Verification items for the finished model (mm, model axes). Face numbers are marked on the shaded views. A direction names the side the tool comes from. Coordinates: 2 decimals unless noted, no trailing zeros. Order: outer loops, then holes, each group sorted by start corner. A loop starts at its lowest first (then second) coordinate and runs counter-clockwise, first axis right, second up.
Q1. Thickness scan on line 1 (Z direction, x = 14, y = 31.5); line 2 (Y direction, x = 5.5, z = -31); line 3 (Z direction, x = 36, y = -1). Record the ranges inside material, lowest first.
Q2. Set-up check for the marked faces 4 and 5: record each of +Z, -Z, +X, -X, +Y, -Y from which the full face is reachable in a straight line by a thin tool's end or side.
Q3. Draft check along Y on the marked faces 1, 2 and 3. Enter one of: pulls with the +Y half, pulls with the -Y half, needs draft (parallel to the pull), parting line crosses it, or undercut.
Q4. Depth check by flat-ended pin: P1, Ø4.5, axis at x = 2.5, z = -9.5, coming from the +Y side; P2, Ø3, axis at x = 26.5, z = 12.5, coming from the +Y side; P3, Ø4, axis at y = 28.5, z = 12.5, coming from the +X side. Enter the tip coordinate at first touch or a pass-through.
Q5. Cross-section at A-A, the plane z = -4. Record the boundary of the cut face in (x, y).
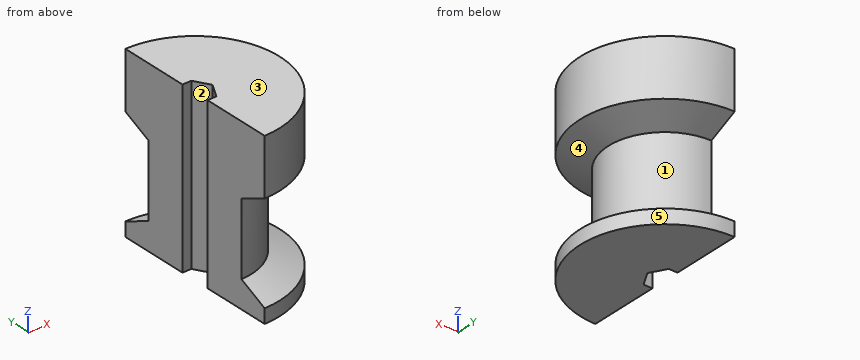
Autodesk Inventor part; units mm, degrees
ref_plane "YZ Plane" through (0, 0, 0) normal (1, 0, 0) x (0, 1, 0)
ref_plane "XZ Plane" through (0, 0, 0) normal (0, 1, 0) x (-1, 0, 0)
ref_plane "XY Plane" through (0, 0, 0) normal (0, 0, 1) x (1, 0, 0)
sketch "Sketch1" plane through (0, 0, 0) normal (0, 0, 1) x (1, 0, 0)
  circle A0 centre (0, 0) radius 25.4
  line L0 (7.9189, 0) -> (3.9595, -6.858)
  line L1 (3.9595, -6.858) -> (-3.9595, -6.858)
  line L2 (-3.9595, -6.858) -> (-7.9189, 0)
  line L3 (-7.9189, 0) -> (-3.9595, 6.858)
  line L4 (-3.9595, 6.858) -> (3.9595, 6.858)
  line L5 (3.9595, 6.858) -> (7.9189, 0)
  dimension "d0" = 50.8
  dimension "d1" = 13.716
extrude "Extrusion1" add sketch "Sketch1" along normal mid plane 76.2
sketch "Sketch3" plane through (0, 0, 0) normal (1, 0, 0) x (0, 1, 0)
  line L0 (25.4, 38.1) -> (-25.4, 38.1)
  line L1 (25.4, 38.1) -> (38.1, 38.1)
  line L2 (25.4, -38.1) -> (25.4, 38.1)
  line L3 (0, -53.34) -> (0, 53.34)
  line L4 (38.1, 38.1) -> (38.1, 12.7)
  line L5 (38.1, 12.7) -> (24.2886, 6.2597)
  line L6 (24.2886, 6.2597) -> (25.4, 6.7779)
  line L7 (25.4, -38.1) -> (25.4, 38.1)
  point P0 (0, 0)
  point P1 (25.4, 19.4779)
  point P2 (25.4, 6.7779)
  dimension "d9" = 12.7
  dimension "d12" = 25.4
  dimension "d13" = 115
revolve "Revolution1" add sketch "Sketch3" angle 360 about axis through (0, 0, -10) along (0, 0, 1)
sketch "Sketch4" plane through (0, 0, 0) normal (1, 0, 0) x (0, 1, 0)
  line L0 (25.4, -38.1) -> (25.4, 6.7779)
  line L1 (-25.4, -38.1) -> (25.4, -38.1)
  line L2 (25.4, -38.1) -> (38.1, -38.1)
  line L3 (38.1, -38.1) -> (38.1, -31.75)
  line L4 (38.1, -31.75) -> (24.8707, -25.5811)
  line L5 (0, -46.9275) -> (0, 14.8652)
  line L6 (24.8707, -25.5811) -> (25.4, -25.8279)
  line L7 (25.4, -38.1) -> (25.4, 6.7779)
  point P0 (0, 0)
  point P1 (25.4, -25.8279)
  dimension "d14" = 12.7
  dimension "d15" = 6.35
  dimension "d16" = 115
revolve "Revolution2" add sketch "Sketch4" angle 360 about axis through (0, 0, -10) along (0, 0, 1)
split "Split1" plane through (0, 0, 0) removes the side toward (-1, 0, 0)
properties part number "pulleyOneHalf"
Check values:
1. line 1: z = -38.1 to -30.06, 11.01 to 38.1
1. line 2: y = -36.07 to -4.19, 4.19 to 36.07
1. line 3: z = -38.1 to -30.78, 11.73 to 38.1
2. face 4: +X
2. face 5: +Z, -Z, +X
3. face 1: parting line crosses it
3. face 2: undercut
3. face 3: needs draft
4. P1: stops at y = 25.4
4. P2: stops at y = 28.74
4. P3: stops at x = 27.36
5. outline: (0, -25.4) arc R25.4 ccw to (0, 25.4) - (0, 6.86) - (3.96, 6.86) - (7.92, 0) - (3.96, -6.86) - (0, -6.86) - close
